from build123d import *

# Parameters (mm, degrees)
SKETCH1_W           = 100
SKETCH1_H           = 100
BOSS_EXTRUDE1_DEPTH = 2.54
FILLET1_R           = 2
CUT_EXTRUDE1_DEPTH  = 10
SKETCH2_R           = 1
CUT_EXTRUDE2_DEPTH  = 10
FILLET2_R           = 10
FILLET3_R           = 5


with BuildPart() as part:
    # Sketch1 → Boss-Extrude1 (new body)
    with BuildSketch(Plane.XZ):
        Rectangle(SKETCH1_W, SKETCH1_H)
    extrude(amount=-BOSS_EXTRUDE1_DEPTH)

    # Fillet1
    fillet1_edges = [part.edges().sort_by_distance(p)[0] for p in [
        (-50, 1.27, 50),
        (50, 1.27, 50),
        (50, 1.27, -50),
        (-50, 1.27, -50),
    ]]
    fillet(fillet1_edges, radius=FILLET1_R)

    # Sketch5 → Cut-Extrude1 (cut)
    with BuildSketch(Plane(origin=(0, 2.54, 0), x_dir=(1, 0, 0), z_dir=(0, 1, 0))):
        with BuildLine():
            Line((-10.582420377, 8.15726173), (-44.633181304, 14.898200311))
            Line((-44.633181304, 14.898200311), (-44.633181304, -28.266598236))
            ThreePointArc((-44.633181304, -28.266598236), (-42.544556917, -30.942665333), (-39.296225546, -29.95674939))
            Line((-39.296225546, -29.95674939), (-33.420366711, -22.611976162))
            ThreePointArc((-33.420366711, -22.611976162), (-41.143464147, -5.184990934), (-22.44623806, -8.89440932))
            Line((-22.44623806, -8.89440932), (-10.025095622, 6.631912364))
            ThreePointArc((-10.025095622, 6.631912364), (-10.331945682, 7.384287968), (-10.582420377, 8.15726173))
        make_face()
        with BuildLine():
            Line((34.336383268, -39.764732741), (2.216428403, 0.384935794))
            ThreePointArc((2.216428403, 0.384935794), (0, 0.159324182), (-2.216428403, 0.384935794))
            Line((-2.216428403, 0.384935794), (-34.336383268, -39.764732741))
            ThreePointArc((-34.336383268, -39.764732741), (-34.697694983, -42.938387386), (-31.993783102, -44.638825712))
            Line((-31.993783102, -44.638825712), (31.993783102, -44.638825712))
            ThreePointArc((31.993783102, -44.638825712), (34.697694983, -42.938387386), (34.336383268, -39.764732741))
        make_face()
        with BuildLine():
            Line((39.838812559, 34.788749055), (10.83835688, 13.038158963))
            ThreePointArc((10.83835688, 13.038158963), (10.959514717, 12.102211852), (11, 11.159324182))
            ThreePointArc((11, 11.159324182), (10.75351226, 8.843730505), (10.025095622, 6.631912364))
            Line((10.025095622, 6.631912364), (39.296225546, -29.95674939))
            ThreePointArc((39.296225546, -29.95674939), (42.631851266, -30.913539718), (44.638825712, -28.08265642))
            Line((44.638825712, -28.08265642), (44.638825712, 32.38875892))
            ThreePointArc((44.638825712, 32.38875892), (42.980459146, 35.072044169), (39.838812559, 34.788749055))
        make_face()
        with BuildLine():
            Line((27.305635475, 44.638825712), (-34.363291806, 44.638825712))
            Line((-34.363291806, 44.638825712), (-44.633181304, 44.638825712))
            Line((-44.633181304, 44.638825712), (-44.633181304, 34.358849433))
            Line((-44.633181304, 34.358849433), (-44.633181304, 25.087137554))
            Line((-44.633181304, 25.087137554), (-8.643933661, 17.962441914))
            ThreePointArc((-8.643933661, 17.962441914), (-2.446557859, 21.883798745), (4.838313038, 21.038126081))
            Line((4.838313038, 21.038126081), (29.105648628, 39.238835577))
            ThreePointArc((29.105648628, 39.238835577), (30.15168277, 42.587516809), (27.305635475, 44.638825712))
        make_face()
        with BuildLine():
            Line((-33.420366711, -22.611976162), (-22.44623806, -8.89440932))
            ThreePointArc((-22.44623806, -8.89440932), (-41.143464147, -5.184990934), (-33.420366711, -22.611976162))
        make_face()
        with BuildLine():
            ThreePointArc((-22.01893977, -11.893547741), (-22.12630101, -10.378835302), (-22.44623806, -8.89440932))
            Line((-22.44623806, -8.89440932), (-33.420366711, -22.611976162))
            ThreePointArc((-33.420366711, -22.611976162), (-25.402259154, -19.71782477), (-22.01893977, -11.893547741))
        make_face()
    extrude(amount=-CUT_EXTRUDE1_DEPTH, mode=Mode.SUBTRACT)

    # Sketch2 → Cut-Extrude2 (cut)
    with BuildSketch(Plane(origin=(0, 2.54, 0), x_dir=(1, 0, 0), z_dir=(0, 1, 0))):
        with Locations(Location((-46.23, -47.5, 0), (0, 0, 90))):
            Circle(SKETCH2_R)
        with Locations(Location((-46.23, 47.5, 0), (0, 0, 90))):
            Circle(SKETCH2_R)
        with Locations(Location((46.23, 47.5, 0), (0, 0, 270))):
            Circle(SKETCH2_R)
        with Locations(Location((46.23, -47.5, 0), (0, 0, 270))):
            Circle(SKETCH2_R)
    extrude(amount=-CUT_EXTRUDE2_DEPTH, mode=Mode.SUBTRACT)

    # Fillet2
    # the kernel refuses this fillet: 10 mm, written as the material it adds along each edge
    with BuildSketch(Plane(origin=(-2.216428403, 2.54, -0.384935794), x_dir=(0.9991591303691161, 0, 0.04100039268143086), z_dir=(0, -1, 0)), Plane(origin=(-10.582420377, 2.54, -8.15726173), x_dir=(0.42439359901934914, 0, 0.9054778148090675), z_dir=(0, -1, 0))) as fillet2_piece_1:
        with BuildLine():
            CenterArc((5.15726697, 9.869275424), FILLET2_R, 216.310191596, 44.415308597)
            Line((-2.90096267, 3.94771017), (0, 0))
            ThreePointArc((0, 0), (1.772810521, 0.143797033), (3.545621042, 0))
        make_face()
    extrude(amount=2.54)
    with BuildSketch(Plane(origin=(2.216428403, 2.54, -0.384935794), x_dir=(0.6246976569815567, 0, 0.780866721894174), z_dir=(0, -1, 0)), Plane(origin=(10.83835688, 2.54, -13.038158963), x_dir=(0.7999967117807752, 0, -0.6000043842672711), z_dir=(0, -1, 0)), Plane(origin=(-10.025095622, 2.54, -6.631912364), x_dir=(-0.624697656981556, 0, 0.7808667218941745), z_dir=(0, -1, 0))) as fillet2_piece_2:
        with BuildLine():
            CenterArc((4.898979486, 10), FILLET2_R, 225.584691403, 44.415308597)
            ThreePointArc((-2.099562637, 2.857142857), (-0.933906367, 1.51372178), (0, 0))
            Line((0, 0), (4.898979486, 0))
        make_face()
    extrude(amount=2.54)
    with BuildSketch(Plane(origin=(4.838313038, 2.54, -21.038126081), x_dir=(0.7999967117807896, 0, -0.600004384267252), z_dir=(0, -1, 0)), Plane(origin=(10.025095622, 2.54, -6.631912364), x_dir=(0.6246976569815559, 0, 0.7808667218941746), z_dir=(0, -1, 0))) as fillet2_piece_3:
        with BuildLine():
            CenterArc((4.898979486, -10), FILLET2_R, 90, 44.415308597)
            ThreePointArc((-2.099562637, -2.857142857), (-0.933906367, -1.51372178), (0, 0))
            Line((0, 0), (4.898979486, 0))
        make_face()
    extrude(amount=2.54)
    with BuildSketch(Plane(origin=(-8.643933661, 2.54, -17.962441914), x_dir=(0.7370833881406508, 0, -0.6758018044716206), z_dir=(0, -1, 0))) as fillet2_piece_4:
        with BuildLine():
            CenterArc((5.159972861, -9.869137303), FILLET2_R, 99.279408895, 44.434942373)
            Line((-2.900792564, -3.951024364), (0, 0))
            ThreePointArc((0, 0), (1.773740671, -0.143948967), (3.547481342, 0))
        make_face()
    extrude(amount=2.54)
    with BuildSketch(Plane(origin=(-44.633181304, 2.54, -25.087137554), x_dir=(0.9809622556130392, 0, 0.19419848882671173), z_dir=(0, -1, 0))) as fillet2_piece_5:
        with BuildLine():
            CenterArc((FILLET2_R * 0.821439873515, -FILLET2_R), FILLET2_R, 90, 78.802094649)
            Line((-FILLET2_R * 0.159522382099, -FILLET2_R * 0.805801511173), (0, 0))
            Line((0, 0), (FILLET2_R * 0.821439873515, 0))
        make_face()
    extrude(amount=2.54)
    with BuildSketch(Plane(origin=(-44.633181304, 2.54, -44.638825712), x_dir=(1, 0, 0), z_dir=(0, -1, 0))) as fillet2_piece_6:
        with BuildLine():
            CenterArc((FILLET2_R, FILLET2_R), FILLET2_R, 180, 90)
            Line((0, FILLET2_R), (0, 0))
            Line((0, 0), (FILLET2_R, 0))
        make_face()
    extrude(amount=2.54)
    with BuildSketch(Plane(origin=(-44.633181304, 2.54, -14.898200311), x_dir=(0.9809622556130391, 0, 0.19419848882671228), z_dir=(0, -1, 0))) as fillet2_piece_7:
        with BuildLine():
            CenterArc((FILLET2_R * 1.21737455442, FILLET2_R), FILLET2_R, 168.802094649, 101.197905351)
            Line((FILLET2_R * 0.236412298804, FILLET2_R * 1.19419848883), (0, 0))
            Line((0, 0), (FILLET2_R * 1.21737455442, 0))
        make_face()
    extrude(amount=2.54)

    # Fillet3
    fillet3_edges = [part.edges().sort_by_distance(p)[0] for p in [
        (0, 1.27, 0.013314064),
        (-11.084977947, 1.27, -7.109148691),
    ]]
    fillet(fillet3_edges, radius=FILLET3_R)


solid = part.part
Build history of the part. All positions in model axes, mm. A direction names the side the tool comes from. Round coordinates to 2 decimals unless told otherwise and drop trailing zeros. Write each loop counter-clockwise with the first axis right and the second up, starting at its lowest first coordinate (ties: lowest second). Pieces come first, ordered by that corner, then holes. Notation, with made-up numbers: (55, 86.5) -> (70, 86.5) arc R20 cw to (70, 106.5) -> close; hole circle Ø2 at (6, 11). An arc over 180 degrees is marked (long way). Use one line per item in the form item = value.
Q1. Band-saw the part on B-B, the plane x = -38. Write the cut outline in (y, z).
Conclusion:
outline = (0, -50) -> (2.54, -50) -> (2.54, -44.06) -> (0, -44.06) -> close; (0, -23.89) -> (2.54, -23.89) -> (2.54, -12.14) -> (0, -12.14) -> close; (0, 28.34) -> (2.54, 28.34) -> (2.54, 50) -> (0, 50) -> close
Q2. Band-saw the part on D-D, the plane z = -8. State how many separate pieces and enclosed holes the cut face has, then the cut area to 3 significant figures.
Conclusion:
separate_pieces = 3
enclosed_holes = 0
area = 95.7 mm²
Q3. Two-plate mould, pull along X, no slides. Class faces 1 (the cylindrical face through (-4.03, 1.29, 2.14)), 2 (the flat face through (-1, 1, 50)), 3 (the flat face through (-50, 1, -1)): released by +X, released by -X, zero draft, split by the parting line, or undercut.
Conclusion:
face_1 = undercut
face_2 = zero draft
face_3 = released by -X
Q4. Band-saw the part on A-A, the plane x = 23.5. Write the cut outline in (y, z).
Conclusion:
outline = (0, -50) -> (2.54, -50) -> (2.54, -44.64) -> (0, -44.64) -> close; (0, -35.03) -> (2.54, -35.03) -> (2.54, -22.53) -> (0, -22.53) -> close; (0, 10.21) -> (2.54, 10.21) -> (2.54, 26.22) -> (0, 26.22) -> close; (0, 44.64) -> (2.54, 44.64) -> (2.54, 50) -> (0, 50) -> close
Q5. Drill centre lines: L1, parallel to X at y = 1.5, z = 47.5; L2, parallel to Z at x = -46.23, y = 2.05; L3, parallel to Z at x = -43, y = 1.9. Where is each one in solid material? Low to high.
Conclusion:
L1 = -50 to -47.23, -45.23 to 45.23, 47.23 to 50
L2 = -50 to -48.5, -46.5 to 46.5, 48.5 to 50
L3 = -50 to -40.12, -27.82 to -8.2, 30.76 to 50
Q6. Band-saw the part on C-C, the plane x = 37. Write the cut outline in (y, z), then the cut area to 3 significant figures.
Conclusion:
outline = (0, -50) -> (2.54, -50) -> (2.54, -32.66) -> (0, -32.66) -> close; (0, 27.09) -> (2.54, 27.09) -> (2.54, 50) -> (0, 50) -> close
area = 102 mm²
Q7. Tool access for faces 4 (the flat face through (0, 2.54, 0)), 5 (the cylindrical face through (-42.593, 1.288, 30.927)): list every direction of +Z, -Z, +X, -X, +Y, -Y with a clear straight run to the whole face (end or side of a thin tool).
Conclusion:
face_4 = +Z, -Z, +X, -X, +Y
face_5 = +Y, -Y
Q8. Drop a flat-ended pin along its axis: P1, Ø1.6, axis at x = 46.23, z = -47.5, coming from the +Y side. Give the stop position or say it passes through.
Conclusion:
P1 = through
